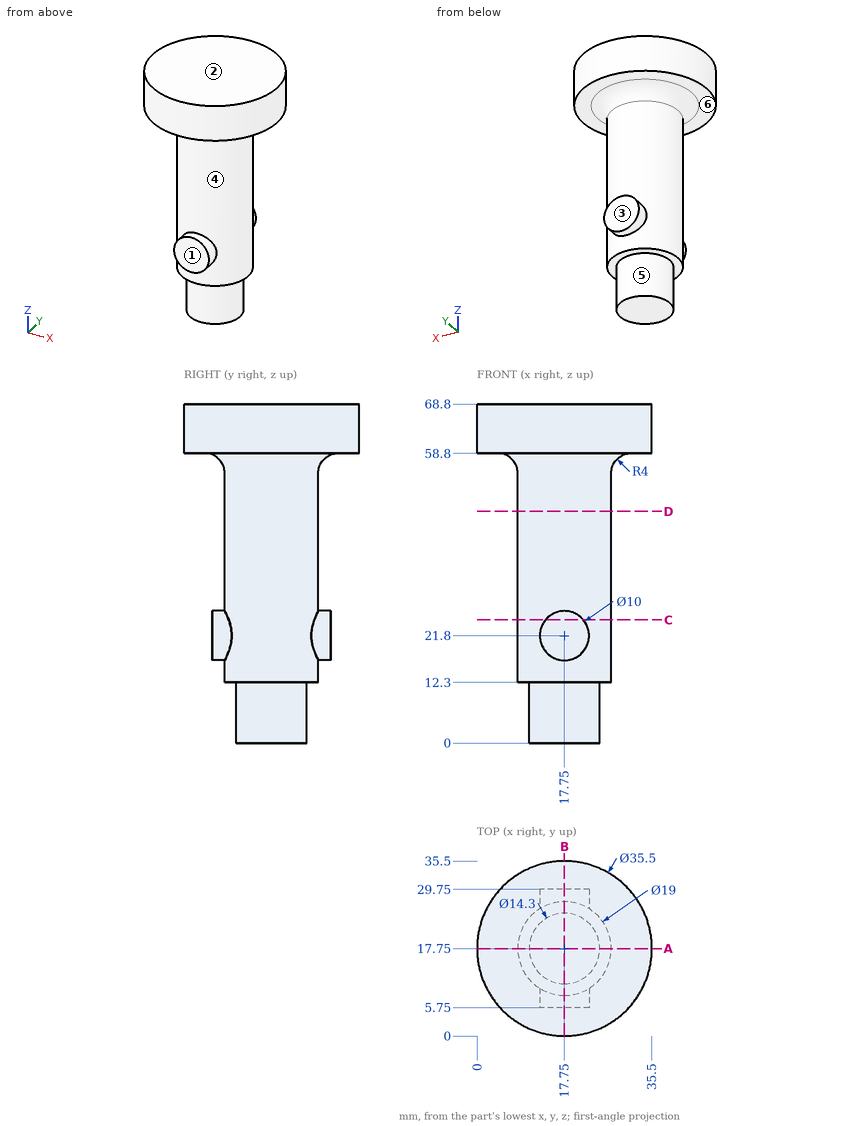
Print and shaded views of the part. All mm, measured from the part's lowest x, y and z. A direction names the side the tool comes from. Coordinates: 2 decimals unless noted, no trailing zeros. Loops run counter-clockwise (first coordinate to the right, second up) from the corner with the lowest first, then second, coordinate; pieces in that order, holes last. Notation, with made-up numbers: (-29, -11) -> (-4, -11) arc R12 cw to (-4, 9) -> close; hole circle Ø11 at (56.25, -1). An arc over 180 degrees is marked (long way). Use a Markdown table: item, result. Add a question column.
Item 1: Band-saw the part on A-A on y = 17.75. Write the cut outline in (x, z), plus the area to 3 significant figures.
Item 2: Which spindle directions (+Z, -Z, +X, -X, +Y, -Y) get a long thin tool onto all of the face, cutting with end or side? Do the marked faces 1, 2 and 3. Say none if no direction does.
Item 3: Flat gauge pins, fed straight in: P1, Ø10, axis at x = 6.5, z = 34.5, coming from the +Y side; P2, Ø10, axis at x = 17, z = 35.5, coming from the +Y side; P3, Ø8, axis at y = 7, z = 16, coming from the +X side. Where does each tip first touch, or does it go through?
Item 4: Band-saw the part on B-B on x = 17.75. Write the cut outline in (y, z).
Item 5: Probe probe 1 along Y at (x, z) = (21.5, 24); probe 2 along Z at (x, y) = (22.5, 11); probe 3 along Z at (x, y) = (26.5, 32). List the from-to ranges inside material, lowest first.
Item 6: Pull direction Z, two halves, no side cores. Call the marked faces 4, 5 and 6: +Z half, -Z half, draft (parallel to the pull), parting line (faces both ways), or undercut.
Item 7: Band-saw the part on D-D on z = 47. Write the cut outline in (x, y).
Item 8: Band-saw the part on C-C on z = 25. Write the cut outline in (x, y).
Geometry says:
| question | item | result |
|---|---|---|
| 1 | outline | (0, 58.8) -> (4.25, 58.8) arc R4 cw to (8.25, 54.8) -> (8.25, 12.3) -> (10.6, 12.3) -> (10.6, 0) -> (24.9, 0) -> (24.9, 12.3) -> (27.25, 12.3) -> (27.25, 54.8) arc R4 cw to (31.25, 58.8) -> (35.5, 58.8) -> (35.5, 68.8) -> (0, 68.8) -> close |
| 1 | area | 1,420 mm² |
| 2 | face 1 | -Z, +X, -X, -Y |
| 2 | face 2 | +Z, +X, -X, +Y, -Y |
| 2 | face 3 | -Z, +X, -X, +Y |
| 3 | P1 | y = 24.9 |
| 3 | P2 | y = 27.25 |
| 3 | P3 | x = 24.43 |
| 4 | outline | (0, 58.8) -> (4.25, 58.8) arc R4 cw to (8.25, 54.8) -> (8.25, 26.8) -> (5.75, 26.8) -> (5.75, 16.8) -> (8.25, 16.8) -> (8.25, 12.3) -> (10.6, 12.3) -> (10.6, 0) -> (24.9, 0) -> (24.9, 12.3) -> (27.25, 12.3) -> (27.25, 16.8) -> (29.75, 16.8) -> (29.75, 26.8) -> (27.25, 26.8) -> (27.25, 54.8) arc R4 cw to (31.25, 58.8) -> (35.5, 58.8) -> (35.5, 68.8) -> (0, 68.8) -> close |
| 5 | probe 1 | 5.75 to 29.75 |
| 5 | probe 2 | 12.3 to 68.8 |
| 5 | probe 3 | 58.8 to 68.8 |
| 6 | face 4 | undercut |
| 6 | face 5 | draft |
| 6 | face 6 | -Z half |
| 7 | outline | circle Ø19 at (17.75, 17.75) |
| 8 | outline | (13.91, 5.75) -> (21.59, 5.75) -> (21.59, 9.06) arc R9.5 ccw to (21.59, 26.44) -> (21.59, 29.75) -> (13.91, 29.75) -> (13.91, 26.44) arc R9.5 ccw to (13.91, 9.06) -> close |
